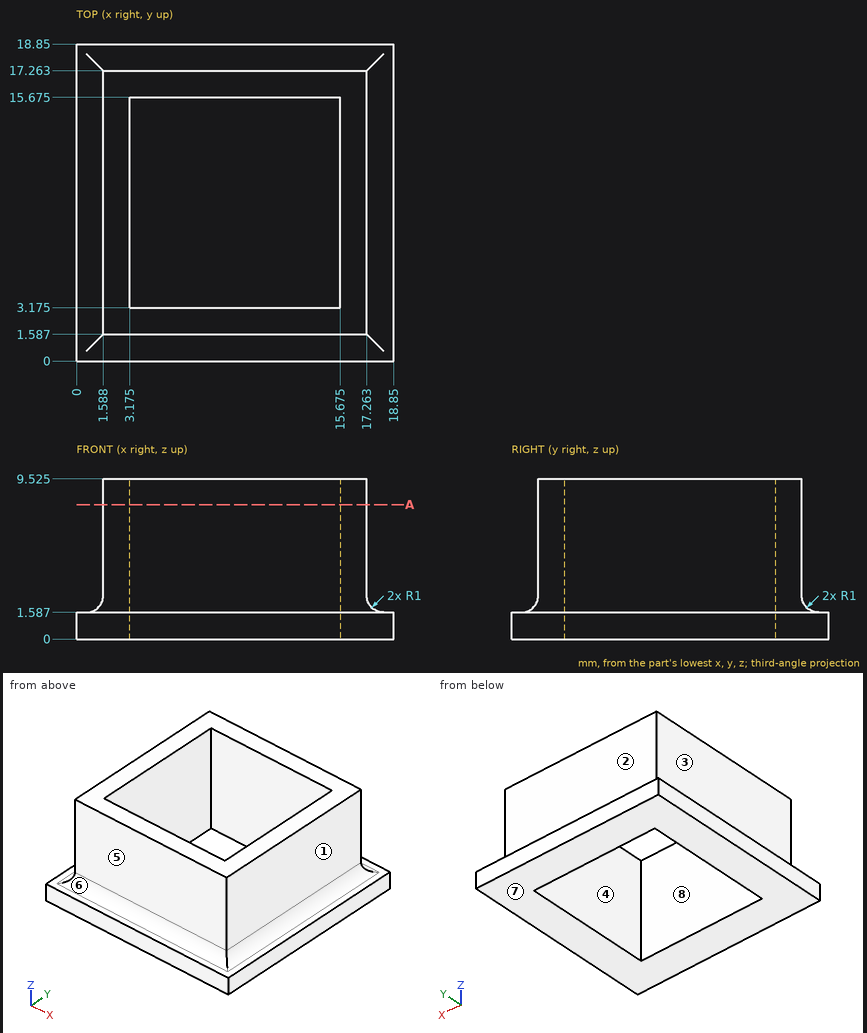
The figure shows three views and two pictorial views of one solid part (mm, origin at its lowest corner). Answer the questions. A direction names the side the tool comes from. Round coordinates to 2 decimals unless told otherwise and drop trailing zeros. Order: outer loops, then holes, each group sorted by start corner. A loop starts at its lowest first (then second) coordinate and runs counter-clockwise, first axis right, second up. Notation, with made-up numbers: (-27.75, 3.25) - (12.25, 3.25) arc R38 ccw to (12.25, 41.25) - close; hole circle Ø5 at (-7.5, 68). An arc over 180 degrees is marked (long way). Write item = value, one per line. Start each with the question number.
1) For a pull along Y with two mould halves and no side action, classify the marked faces 6, 7 and 8 as released by +Y, released by -Y, zero draft, split by the parting line, or undercut.
2) Given pin 1 (5.5 mm diameter, centred on x = 8.5, z = 6, fed in from +Y); pin 2 (4 mm diameter, centred on y = 4, z = 2.5, fed in from -X); pin 3 (5 mm diameter, centred on y = 9, z = 4.5, fed in from -X); pin 4 (1.5 mm diameter, centred on x = 6.5, z = 6, fed in from -Y), each flat-ended and moving along its own axis, determine where each tip first touches the part or whether it passes through.
3) Straight lines are drawn through the part: L1, parallel to Y at x = 10.5, z = 4.75 (1 decimal); L2, parallel to X at y = 15.75, z = 9. For each, find the intervals that lie inside material, in ascending order.
4) For the marked faces 1, 2, 3, 4 and 5, determine the directions among +Z, -Z, +X, -X, +Y, -Y from which every point of the face is accessible in a straight line to the end or side of a thin tool.
5) Section A-A, the plane z = 8 is taken. Write down the section's boundary in (x, y) (1 decimal).
Results list:
q1.face_6 = released by -Y
q1.face_7 = zero draft
q1.face_8 = undercut
q2.pin_1 = 17.26
q2.pin_2 = 0
q2.pin_3 = 1.4
q2.pin_4 = 1.59
q3.L1 = 1.6 to 3.2, 15.7 to 17.3
q3.L2 = 1.59 to 17.26
q4.face_1 = +Z, +X, +Y, -Y
q4.face_2 = +Z, +X, -X, +Y
q4.face_3 = +Z, -X, +Y, -Y
q4.face_4 = +Z, -Z
q4.face_5 = +Z, +X, -X, -Y
q5.outline = (1.6, 1.6) - (17.3, 1.6) - (17.3, 17.3) - (1.6, 17.3) - close; hole (3.2, 3.2) - (15.7, 3.2) - (15.7, 15.7) - (3.2, 15.7) - close
